from build123d import *

# Parameters (mm, degrees)
F1_DEPTH = 12
F3_DEPTH = 25
F5_DEPTH = 25


with BuildPart() as f1:
    # F0 (on Front) → F1 (new body)
    with BuildSketch(Plane.XZ):
        Polygon((0, 2), (0, 0), (6, 0), (6, 2), (4, 2), (4, 6), (4.5, 6), (4.5, 10), (1.5, 10), (1.5, 6), (2, 6), (2, 2), align=None)
    extrude(amount=F1_DEPTH)

    # F2 (on face) → F3 (cut)
    with BuildSketch(Plane(origin=(0, 0, 0), x_dir=(0, -1, 0), z_dir=(-1, 0, 0))):
        with BuildLine():
            Line((6, 6.23), (6, 0))
            Line((6, 0), (13.765802, 0))
            Line((13.765802, 0), (13.765802, 10.684827))
            Line((13.765802, 10.684827), (0, 10.684827))
            Line((0, 10.684827), (0, 10))
            Line((0, 10), (1, 10))
            Line((1, 10), (1, 9.5))
            Line((1, 9.5), (1.75, 9.5))
            Line((1.75, 9.5), (1.75, 10))
            Line((1.75, 10), (2.525424, 10))
            Line((2.525424, 10), (11.041579, 6.674281))
            ThreePointArc((11.041579, 6.674281), (11.165583, 6.452114), (10.971159, 6.287997))
            Line((10.971159, 6.287997), (6, 6.23))
        make_face()
    extrude(amount=-F3_DEPTH, mode=Mode.SUBTRACT)

    # F4 (on face) → F5 (cut)
    with BuildSketch(Plane(origin=(0, 0, 0), x_dir=(1, 0, 0), z_dir=(0, 0, -1))):
        with BuildLine():
            ThreePointArc((3.5, 11.886248), (3, 12.386248), (2.5, 11.886248))
            Line((2.5, 11.886248), (2.5, 7.971159))
            ThreePointArc((2.5, 7.971159), (3, 7.471159), (3.5, 7.971159))
            Line((3.5, 7.971159), (3.5, 11.886248))
        make_face()
    extrude(amount=-F5_DEPTH, mode=Mode.SUBTRACT)


solid = f1.part
Design review of the part built by this model. Coordinates are the model's own, in mm. A direction names the side the tool comes from. Give positions to 0.01 mm unless a question says otherwise; leave off trailing zeros. Loops run counter-clockwise (first coordinate to the right, second up) from the corner with the lowest first, then second, coordinate; pieces in that order, holes last. Notation, with made-up numbers: M 75.5,2 L 109.5,2 A24 ccw 109.5,22 Z; hole C 76,-4 d2. An arc over 180 degrees is marked long. One line per question, with ' | ' between items. Start each with the question number.
1. To check wall thickness, follow L1, parallel to Z at x = 1.6, y = -2.5; L2, parallel to X at y = -4.5, z = 3.75; L3, parallel to X at y = -5.5, z = 8.75. State the ranges of each line that lie inside material, in increasing order.
2. Add section A-A (x = 3). Write out the cut boundary in (y, z), plus the area to 3 significant figures.
3. Insertion check: P1, Ø4.5, axis at y = -6.5, z = 8, coming from the -X side; P2, Ø1.5, axis at y = -4.5, z = 8.5, coming from the +X side; P3, Ø1.2, axis at y = -3.5, z = 3, coming from the -X side. Each pin has a flat end and moves straight along its axis. Give the tip position at first contact, or say it passes through.
4. For faces 1 (the face through (4, -3, 4)), 2 (the face through (2, -3, 4)), 3 (the face through (3, -6, 2)), 4 (the face through (3.5, -9, 7)), 5 (the face through (4.5, -4, 8)), list the 3-axis set-ups (+Z, -Z, +X, -X, +Y, -Y) from which the entire face can be reached by the end or side of a thin tool; tool diameter is ignored.
5. Add section B-B (y = -5.25). Write out the cut boundary in (x, z).
6. Add section C-C (z = 5). Write out the cut boundary in (x, y).
7. Add section D-D (x = 5.4). Write out the cut boundary in (y, z), plus the area to 3 significant figures.
Worked out:
1) L1: z = 0 to 2, 6 to 10 | L2: x = 2 to 4 | L3: x = 1.5 to 4.5
2) outline: M -7.47,6.25 L -6,6.23 L -6,0 L 0,0 L 0,10 L -1,10 L -1,9.5 L -1.75,9.5 L -1.75,10 L -2.53,10 L -7.47,8.07 Z | area: 60.4 mm²
3) P1: stops at x = 1.5 | P2: stops at x = 4.5 | P3: stops at x = 2
4) face 1: +X, +Y, -Y | face 2: -X, +Y, -Y | face 3: -Z, +X, -X, -Y | face 4: +Z, -Z, -Y | face 5: +Z, +X, +Y, -Y
5) outline: M 0,0 L 6,0 L 6,2 L 4,2 L 4,6 L 4.5,6 L 4.5,8.94 L 1.5,8.94 L 1.5,6 L 2,6 L 2,2 L 0,2 Z
6) outline: M 2,-6 L 4,-6 L 4,0 L 2,0 Z
7) outline: M -6,0 L 0,0 L 0,2 L -6,2 Z | area: 12.0 mm²
